Autodesk Fusion 360 part; units mm, degrees
sketch "Sketch1" plane through (0, 0, 0) normal (0, 0, 1) x (1, 0, 0)
  line L0 (0, 0) -> (40, 0)
  line L1 (40, 0) -> (40, 28)
  line L2 (40, 28) -> (0, 28)
  line L3 (0, 28) -> (0, 0)
  circle A0 centre (20, 14) radius 4.05
  dimension "d1" = 40
  dimension "d2" = 28
  dimension "d3" = 8.1
  dimension "d10" = 14
  dimension "d11" = 20
extrude "Extrude1" add sketch "Sketch1" along normal blind 5
sketch "Sketch2" plane through (0, 0, 5) normal (0, 0, 1) x (-1, 0, 0)
  circle A0 centre (-20, -14) radius 4.05
  line L0 (0, -28) -> (0, 0)
  line L1 (0, 0) -> (-40, 0)
  line L2 (-40, 0) -> (-40, -28)
  line L3 (-40, -28) -> (0, -28)
  line L4 (0, -28) -> (-40, -28)
  line L5 (-40, -28) -> (-40, -23)
  line L6 (-40, -23) -> (0, -23)
  line L7 (0, -23) -> (0, -28)
  line L8 (0, 0) -> (-40, 0)
  line L9 (-40, 0) -> (-40, -5)
  line L10 (-40, -5) -> (0, -5)
  line L11 (0, -5) -> (0, 0)
  dimension "d6" = 40
  dimension "d7" = 5
  dimension "d8" = 40
  dimension "d9" = 5
extrude "Extrude2" add sketch "Sketch2" along normal blind 10 contours L0 L2 L3 L4 L5 L6 L7 | L0 L1 L2 L8 L9 L10 L11
chamfer "Chamfer1" distance 1 angle 45 2 edges at (20, 23, 15) (20, 5, 15)
sketch "Sketch3" plane through (0, 0, 0) normal (0, 0, 1) x (1, 0, 0)
  circle A0 centre (20, 14) radius 6
  circle A1 centre (20, 14) radius 4.05
  dimension "d15" = 12
extrude "Extrude3" add sketch "Sketch3" against normal blind 5
Part model, mm, in its own coordinate system. A direction names the side the tool comes from. Round coordinates to 2 decimals unless told otherwise and drop trailing zeros. Order: outer loops, then holes, each group sorted by start corner. A loop starts at its lowest first (then second) coordinate and runs counter-clockwise, first axis right, second up. Notation, with made-up numbers: M 40.25,16.25 L 66.25,16.25 A18 cw 66.25,45.25 Z; hole C -9,86.5 d4. An arc over 180 degrees is marked long. Answer in a Markdown table with one row per item. Add a question column.
Q1. Cut at A-A on z = 7.25. Give the cut face in (x, y), and give its area (3 significant figures).
Q2. Cut at C-C on x = 20. Give the cut face in (y, z), and give its area (3 significant figures).
Q3. 3-axis set-ups, long thin cutter, end or side, ignore diameter. For faces 1 (the face through (19.7, 20.4, 0)), 2 (the face through (16.786, 16.464, -0.07)), 3 (the face through (24.2, 14.1, 5)): which of +Z, -Z, +X, -X, +Y, -Y reach the whole face in a straight line?
Q4. Cut at B-B on y = 14. Give the cut face in (x, z), and give its area (3 significant figures).
Q5. Pin check, flat tips, straight feed: pin 1 (10 mm diameter, centred on x = 25, z = -1, fed in from +Y); pin 2 (1.5 mm diameter, centred on x = 22, z = -2, fed in from -Y); pin 3 (14.5 mm diameter, centred on x = 16, y = 16.5, fed in from +Z); pin 4 (10 mm diameter, centred on x = 10, y = 17.5, fed in from +Z). Stop position of each tip, or through.
Q6. Wall check: L1, parallel to Y at x = 20, z = -0.25; L2, parallel to Y at x = 25, z = 6.25; L3, parallel to Z at x = 5, y = 7. Give the ranges that are in metal, low to high. Write a range as from..to.
Q7. Cut at D-D on z = -3.25. Give the cut face in (x, y), and give its area (3 significant figures).
Q8. Mould opens along Y. For faces 4 (the face through (20, 28, 7)), 5 (the face through (19.7, 23.5, 14.5)), 6 (the face through (25.54, 11.7, -2.46)), 7 (the face through (40, 14, 4)) say: +Y half, -Y half, draft (parallel to the pull), parting line (faces both ways), or undercut.
Established:
| question | item | result |
|---|---|---|
| 1 | outline | M 0,0 L 40,0 L 40,5 L 0,5 Z; M 0,23 L 40,23 L 40,28 L 0,28 Z |
| 1 | area | 400 mm2 |
| 2 | outline | M 0,0 L 8,0 L 8,-5 L 9.95,-5 L 9.95,5 L 5,5 L 5,14 L 4,15 L 0,15 Z; M 18.05,-5 L 20,-5 L 20,0 L 28,0 L 28,15 L 24,15 L 23,14 L 23,5 L 18.05,5 Z |
| 2 | area | 218 mm2 |
| 3 | face 1 | -Z |
| 3 | face 2 | +Z, -Z |
| 3 | face 3 | +Z, +X, -X |
| 4 | outline | M 0,0 L 14,0 L 14,-5 L 15.95,-5 L 15.95,5 L 0,5 Z; M 24.05,-5 L 26,-5 L 26,0 L 40,0 L 40,5 L 24.05,5 Z |
| 4 | area | 179 mm2 |
| 5 | pin 1 | stops at y = 28 |
| 5 | pin 2 | stops at y = 8.13 |
| 5 | pin 3 | stops at z = 14.75 |
| 5 | pin 4 | stops at z = 5 |
| 6 | L1 | y = 8..9.95, 18.05..20 |
| 6 | L2 | y = 0..5, 23..28 |
| 6 | L3 | z = 0..5 |
| 7 | outline | C 20,14 d12; hole C 20,14 d8.1 |
| 7 | area | 61.6 mm2 |
| 8 | face 4 | +Y half |
| 8 | face 5 | undercut |
| 8 | face 6 | parting line |
| 8 | face 7 | draft |
